Design review of the part shown in the three views and the two pictorial views. Dimensions are in mm from the part's minimum x, y and z. Round coordinates to 2 decimals unless told otherwise and drop trailing zeros. Order: outer loops, then holes, each group sorted by start corner. A loop starts at its lowest first (then second) coordinate and runs counter-clockwise, first axis right, second up. Notation, with made-up numbers: M 32.5,-24.5 L 46.5,-24.5 A18 ccw 46.5,-8.5 Z; hole C 16,-18.75 d3. An arc over 180 degrees is marked long. Use a Markdown table: item, result. Add a question column.
(1) Take a section at B-B (x = 28.9). Write out the cut boundary in (y, z).
(2) For pin 1 (6.5 mm diameter, centred on x = 84.5, z = 6.5, fed in from -Y); pin 2 (3 mm diameter, centred on x = 84.5, y = 23.5, fed in from +Z); pin 3 (4 mm diameter, centred on x = 88, z = 9, fed in from +Y); pin 4 (1.5 mm diameter, centred on x = 18, z = 3, fed in from -Y), all flat-tipped, find the tip position at first contact; note any pin that passes through.
(3) To check wall thickness, follow probe 1 along X at (y, z) = (8, 7.5); probe 2 along Z at (x, y) = (86, 8); probe 3 along Z at (x, y) = (6.5, 25). State the ranges of each line that lie inside material, in increasing order. Write a range as from..to.
(4) Take a section at D-D (x = 52). Write out the cut boundary in (y, z).
(5) The part is to be moulded in two halves that separate along Z. For the marked faces 1 and 2, say which applies: released by +Z, released by -Z, zero draft, split by the parting line, or undercut.
(6) Take a section at A-A (z = 7.5). Write out the cut boundary in (x, y).
(7) Take a section at C-C (y = 8). Count the separate pieces of the cut face and the enclosed holes in it, then the cut area to 3 significant figures.
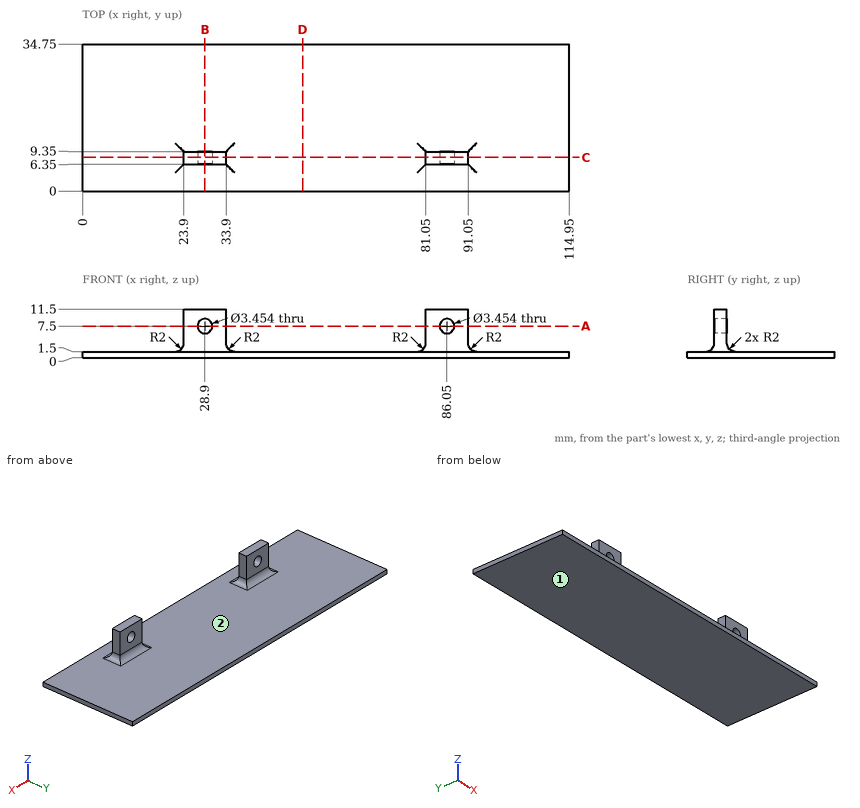
Verdict:
| question | item | result |
|---|---|---|
| 1 | outline | M 0,0 L 34.75,0 L 34.75,1.5 L 11.35,1.5 A2 cw 9.35,3.5 L 9.35,5.77 L 6.35,5.77 L 6.35,3.5 A2 cw 4.35,1.5 L 0,1.5 Z; M 6.35,9.23 L 9.35,9.23 L 9.35,11.5 L 6.35,11.5 Z |
| 2 | pin 1 | stops at y = 6.33 |
| 2 | pin 2 | stops at z = 1.5 |
| 2 | pin 3 | stops at y = 9.35 |
| 2 | pin 4 | passes through |
| 3 | probe 1 | x = 23.9..27.17, 30.63..33.9, 81.05..84.32, 87.78..91.05 |
| 3 | probe 2 | z = 0..5.77, 9.23..11.5 |
| 3 | probe 3 | z = 0..1.5 |
| 4 | outline | M 0,0 L 34.75,0 L 34.75,1.5 L 0,1.5 Z |
| 5 | face 1 | released by -Z |
| 5 | face 2 | released by +Z |
| 6 | outline | M 23.9,6.35 L 27.17,6.35 L 27.17,9.35 L 23.9,9.35 Z; M 30.63,6.35 L 33.9,6.35 L 33.9,9.35 L 30.63,9.35 Z; M 81.05,6.35 L 84.32,6.35 L 84.32,9.35 L 81.05,9.35 Z; M 87.78,6.35 L 91.05,6.35 L 91.05,9.35 L 87.78,9.35 Z |
| 7 | separate pieces | 1 |
| 7 | enclosed holes | 2 |
| 7 | area | 357 mm^2 |
